from build123d import *

# Parameters (mm, degrees)
SKETCH_4_R      = 1.5
EXTRUDE_3_DEPTH = 0.5
EXTRUDE_4_DEPTH = 10
SKETCH_6_W      = 5
SKETCH_6_H      = 0.551688959
EXTRUDE_5_DEPTH = 2


with BuildPart() as part:
    # Эскиз4 → Бобышка-Вытянуть3 (new body)
    with BuildSketch(Plane.XY):
        Polygon((-2, -8.5), (2, -6.634769367), (2, 6), (-2, 6), align=None)
        with Locations((0, 4)):
            Circle(SKETCH_4_R, mode=Mode.SUBTRACT)
    extrude(amount=EXTRUDE_3_DEPTH)

    # Эскиз5 → Бобышка-Вытянуть4 (add)
    with BuildSketch(Plane.XY.offset(0.5)):
        Polygon((-2, -8.5), (2, -6.634769367), (2, -6.083080408), (-2, -7.948311041), align=None)
    extrude(amount=EXTRUDE_4_DEPTH)

    # Эскиз6 → Бобышка-Вытянуть5 (add)
    with BuildSketch(Plane(origin=(2, 0, 0), x_dir=(0, 0, -1), z_dir=(1, 0, 0))):
        with Locations((-8, -6.358924888)):
            Rectangle(SKETCH_6_W, SKETCH_6_H)
    extrude(amount=EXTRUDE_5_DEPTH)


solid = part.part
Geometry check sheet. Reference: the model listing, model coordinates, mm. A direction names the side the tool comes from. Give positions to 0.01 mm unless a question says otherwise; leave off trailing zeros. Order: outer loops, then holes, each group sorted by start corner. A loop starts at its lowest first (then second) coordinate and runs counter-clockwise, first axis right, second up. Notation, with made-up numbers: (-12, 66.5) - (7, 66.5) arc R18 ccw to (7, 72.5) - close; hole circle Ø1 at (42.25, 30). An arc over 180 degrees is marked (long way). Use one line per item in the form item = value.
1) Draft check along Y on faces 1 (the face through (0, -1, 0)), 2 (the face through (0.806, 5.265, 0.246)), 3 (the face through (3, -6.083, 8)). Enter one of: released by +Y, released by -Y, zero draft, split by the parting line, or undercut.
Working result:
face_1 = zero draft
face_2 = undercut
face_3 = released by +Y
2) Material ranges on probe 1 along Z at (x, y) = (-0.3, -6.5); probe 2 along Y at (x, z) = (3.3, 6.75); probe 3 along Y at (x, z) = (0, 0.25), recorded low to high. Write a range as from..to.
Working result:
probe_1 = 0..0.5
probe_2 = -6.63..-6.08
probe_3 = -7.57..2.5, 5.5..6
3) Sectioned sample at B-B (x = 0). Record the boundary of the cut face in (y, z).
Working result:
outline = (-7.57, 0) - (2.5, 0) - (2.5, 0.5) - (-7.02, 0.5) - (-7.02, 10.5) - (-7.57, 10.5) - close; (5.5, 0) - (6, 0) - (6, 0.5) - (5.5, 0.5) - close
4) Depth check by flat-ended pin: pin 1 Ø3 at (x, z) = (0.5, 8.5) entering from -Y; pin 2 Ø1 at (x, z) = (3, 7.5) entering from +Y; pin 3 Ø1.6 at (x, z) = (3.5, 7.5) entering from -Y. Enter the tip coordinate at first touch or a pass-through.
Working result:
pin_1 = -8.03
pin_2 = -6.08
pin_3 = -6.63
5) Access from +Z, -Z, +X, -X, +Y, -Y to the whole of each face (thin tool, end or side, straight path). Record for faces 4 (the face through (-2, -4.4, 0.2)), 5 (the face through (2, -2.2, 0.3)), 6 (the face through (0.03, -7, 5.43)), 7 (the face through (3, -6.635, 8)), 8 (the face through (1, -6.9, 10.5)).
Working result:
face_4 = +Z, -Z, -X, +Y, -Y
face_5 = -Z, +X, +Y, -Y
face_6 = +Z, -X, +Y
face_7 = +Z, -Z, +X, -Y
face_8 = +Z, +X, -X, +Y, -Y
6) Sectioned sample at A-A (y = 4). Record the boundary of the cut face in (x, z).
Working result:
outline = (-2, 0) - (-1.5, 0) - (-1.5, 0.5) - (-2, 0.5) - close; (1.5, 0) - (2, 0) - (2, 0.5) - (1.5, 0.5) - close
7) Sectioned sample at D-D (x = 3.3). Record the boundary of the cut face in (y, z), and give its area (3 significant figures).
Working result:
outline = (-6.63, 5.5) - (-6.08, 5.5) - (-6.08, 10.5) - (-6.63, 10.5) - close
area = 2.76 mm^2
8) Sectioned sample at C-C (z = 9.75). Record the boundary of the cut face in (x, y), and give its area (3 significant figures).
Working result:
outline = (-2, -8.5) - (2, -6.63) - (4, -6.63) - (4, -6.08) - (2, -6.08) - (-2, -7.95) - close
area = 3.31 mm^2
